CAD build for the part. Positions are in the model's coordinates, mm. Face numbers are marked on the shaded views. Give positions to 0.01 mm unless a question says otherwise; leave off trailing zeros. Order: outer loops, then holes, each group sorted by start corner. A loop starts at its lowest first (then second) coordinate and runs counter-clockwise, first axis right, second up. Notation, with made-up numbers: (86.25, 89) -> (123.25, 89) arc R14 cw to (123.25, 114) -> close; hole circle Ø10 at (1.25, -15). An arc over 180 degrees is marked (long way). Use one line per item in the form item = value. Start each with the question number.
1) Probe line 1 (X direction, y = 4.5, z = -1); line 2 (Y direction, x = 5, z = -0.3); line 3 (X direction, y = 8.5, z = -0.4). List the from-to ranges inside material, lowest first.
2) Cut at B-B, the plane y = 4.5. Give the cut face in (x, z).
3) Drop a flat-ended pin along its axis: P1, Ø1.5, axis at x = 45, y = 4.5, coming from the +Z side. Give the stop position or say it passes through.
4) Cut at A-A, the plane x = 5. Give the cut face in (y, z).
5) Cut at C-C, the plane z = -2.3. Give the cut face in (x, y), and give its area (3 significant figures).
6) Mould opens along Y. For the marked faces 1, 2 and 3 say: pulls with the +Y half, pulls with the -Y half, needs draft (parallel to the pull), parting line crosses it, or undercut.
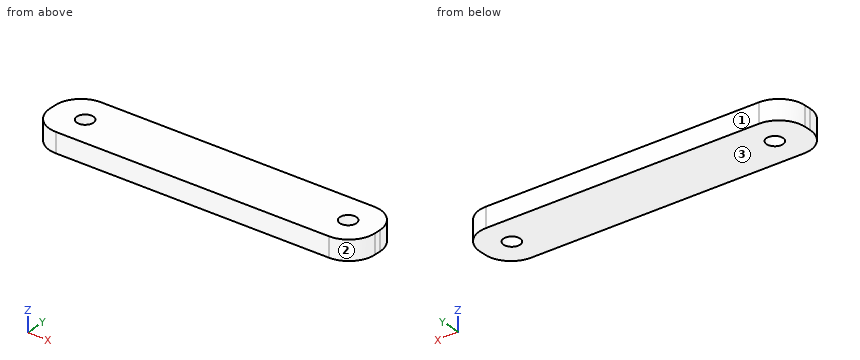
from build123d import *

# Parameters (mm, degrees)
CROQUIS1_W                = 49.5
CROQUIS1_H                = 9
CROQUIS1_R                = 1.25
BRIDA_BASE1_DEPTH         = 3
TALADRO_ROSCADO_M31_D     = 2.5
TALADRO_ROSCADO_M31_DEPTH = 3
REDONDEO1_R               = 4


# Sheet-metal steps are written as plain solids
with BuildPart() as part:
    # Croquis1 → Brida base1 (new body)
    with BuildSketch(Plane.XY):
        with Locations((24.75, 4.5)):
            Rectangle(CROQUIS1_W, CROQUIS1_H)
        with Locations((5, 4.5)):
            Circle(CROQUIS1_R, mode=Mode.SUBTRACT)
        with Locations((45, 4.5)):
            Circle(CROQUIS1_R, mode=Mode.SUBTRACT)
    extrude(amount=-BRIDA_BASE1_DEPTH)

    # Taladro roscado M31
    with Locations(Plane(origin=(5, 4.5, 0), x_dir=(1, 0, 0), z_dir=(0, 0, 1))):
        with Locations((0, 0), (40, 0)):
            Hole(TALADRO_ROSCADO_M31_D / 2, depth=TALADRO_ROSCADO_M31_DEPTH)

    # Redondeo1
    redondeo1_edges = [part.edges().sort_by_distance(p)[0] for p in [
        (0, 9, -1.5),
        (49.5, 9, -1.5),
        (49.5, 0, -1.5),
        (0, 0, -1.5),
    ]]
    fillet(redondeo1_edges, radius=REDONDEO1_R)


solid = part.part
Result:
q1.line_1 = 0 to 3.75, 6.25 to 43.75, 46.25 to 49.5
q1.line_2 = 0 to 3.25, 5.75 to 9
q1.line_3 = 2.06 to 47.44
q2.outline = (0, -3) -> (3.75, -3) -> (3.75, 0) -> (0, 0) -> close; (6.25, -3) -> (43.75, -3) -> (43.75, 0) -> (6.25, 0) -> close; (46.25, -3) -> (49.5, -3) -> (49.5, 0) -> (46.25, 0) -> close
q3.P1 = through
q4.outline = (0, -3) -> (3.25, -3) -> (3.25, 0) -> (0, 0) -> close; (5.75, -3) -> (9, -3) -> (9, 0) -> (5.75, 0) -> close
q5.outline = (0, 4) arc R4 ccw to (4, 0) -> (45.5, 0) arc R4 ccw to (49.5, 4) -> (49.5, 5) arc R4 ccw to (45.5, 9) -> (4, 9) arc R4 ccw to (0, 5) -> close; hole circle Ø2.5 at (5, 4.5); hole circle Ø2.5 at (45, 4.5)
q5.area = 422 mm²
q6.face_1 = pulls with the +Y half
q6.face_2 = pulls with the -Y half
q6.face_3 = needs draft
